Verification items for the finished model (mm, model axes). A direction names the side the tool comes from. Round coordinates to 2 decimals unless told otherwise and drop trailing zeros. Order: outer loops, then holes, each group sorted by start corner. A loop starts at its lowest first (then second) coordinate and runs counter-clockwise, first axis right, second up. Notation, with made-up numbers: (-32.5, 69) -> (8.5, 69) arc R10 cw to (8.5, 73) -> close; hole circle Ø3 at (-26, 28). An arc over 180 degrees is marked (long way). Return JSON: item names as keys, results as strings. Group by question number.
Item 1: Scan lines: probe 1 along X at (y, z) = (2.9, 0); probe 2 along X at (y, z) = (3.75, 16); probe 3 along Z at (x, y) = (-2, 1.6). Record each from-to range of solid material in increasing order. Write a range as from..to.
Item 2: Sectioned sample at C-C on y = 1.95. Record the cut outline in (x, z), plus the area to 3 significant figures.
Item 3: Draft check along Z on faces 1 (the cylindrical face through (-17.15, 2.03, -16.99)), 2 (the cylindrical face through (0.44, 2.03, -10.04)), 3 (the flat face through (20, 2, 3)). Enter one of: pulls with the +Z half, pulls with the -Z half, needs draft (parallel to the pull), parting line crosses it, or undercut.
Item 4: Sectioned sample at B-B on z = 0. Record the cut outline in (x, y).
Item 5: Sectioned sample at A-A on x = 0. Record the cut outline in (y, z), plus the area to 3 significant figures.
Item 6: Sectioned sample at D-D on x = 16. Record the cut outline in (y, z).
Item 7: Access from +Z, -Z, +X, -X, +Y, -Y to the whole of each face (thin tool, end or side, straight path). Record for faces 4 (the flat face through (12.5, 2, 18)), 5 (the flat face through (-12.5, 2, 17)), 6 (the flat face through (0, 2, -20)).
Item 8: Depth check by flat-ended pin: pin 1 Ø1.2 at (x, y) = (17.5, 2) entering from +Z; pin 2 Ø2 at (y, z) = (1.5, 18.5) entering from -X. Enter the tip coordinate at first touch or a pass-through.
```python
from build123d import *

# Parameters (mm, degrees)
EXTRUDE_1_DEPTH     = 4
SKETCH_5_R          = 10.05
CUT_EXTRUDE_4_DEPTH = 29.565713714
FILLET_1_R          = 10


with BuildPart() as part:
    # Эскиз1 → Бобышка-Вытянуть1 (new body)
    with BuildSketch(Plane(origin=(0, 0, 0), x_dir=(1, 0, 0), z_dir=(0, 1, 0))):
        Polygon((-20, -15), (-12.5, -15), (-12.5, -20), (12.5, -20), (12.5, -15), (20, -15), (20, 20), (-20, 20), align=None)
    extrude(amount=EXTRUDE_1_DEPTH)

    # Эскиз5 → Вырез-Вытянуть4 (cut, through all)
    with BuildSketch(Plane(origin=(0, 4, 0), x_dir=(1, 0, 0), z_dir=(0, 1, 0))):
        with Locations(Location((0, 0, 0), (0, 0, 270))):
            Circle(SKETCH_5_R)
    extrude(amount=-CUT_EXTRUDE_4_DEPTH, mode=Mode.SUBTRACT)

    # Скругление1
    fillet_1_edges = [part.edges().sort_by_distance(p)[0] for p in [
        (-20, 2, -20),
        (20, 2, -20),
    ]]
    fillet(fillet_1_edges, radius=FILLET_1_R)


solid = part.part
```
Recorded:
{
 "1": {"probe 1": "-20..-10.05, 10.05..20", "probe 2": "-12.5..12.5", "probe 3": "-20..-9.85, 9.85..20"},
 "2": {"outline": "(-20, -10) arc R10 ccw to (-10, -20) -> (10, -20) arc R10 ccw to (20, -10) -> (20, 15) -> (12.5, 15) -> (12.5, 20) -> (-12.5, 20) -> (-12.5, 15) -> (-20, 15) -> close; hole circle Ø20.1 at (0, 0)", "area": "1,160 mm²"},
 "3": {"face 1": "pulls with the -Z half", "face 2": "undercut", "face 3": "needs draft"},
 "4": {"outline": "(-20, 0) -> (-10.05, 0) -> (-10.05, 4) -> (-20, 4) -> close; (10.05, 0) -> (20, 0) -> (20, 4) -> (10.05, 4) -> close"},
 "5": {"outline": "(0, -20) -> (4, -20) -> (4, -10.05) -> (0, -10.05) -> close; (0, 10.05) -> (4, 10.05) -> (4, 20) -> (0, 20) -> close", "area": "79.6 mm²"},
 "6": {"outline": "(0, -18) -> (4, -18) -> (4, 15) -> (0, 15) -> close"},
 "7": {"face 4": "+Z, +X, +Y, -Y", "face 5": "+Z, -X, +Y, -Y", "face 6": "-Z, +X, -X, +Y, -Y"},
 "8": {"pin 1": "z = 15", "pin 2": "x = -12.5"}
}
